Design review of the part built by this model. Coordinates are the model's own, in mm. A direction names the side the tool comes from. Coordinates: 2 decimals unless noted, no trailing zeros. Order: outer loops, then holes, each group sorted by start corner. A loop starts at its lowest first (then second) coordinate and runs counter-clockwise, first axis right, second up. Notation, with made-up numbers: M 63,56.25 L 71,56.25 A20 ccw 71,94.25 Z; hole C 70.25,2 d3. An arc over 180 degrees is marked long. Use CSV: the item, a comma, the result in double quotes.
```python
from build123d import *

# Parameters (mm, degrees)
BOSS_EXTRUDE1_DEPTH = 5.842
SKETCH2_R           = 2.54
BOSS_EXTRUDE2_DEPTH = 2.54
CUT_EXTRUDE1_REACH  = 37.14
SKETCH3_R           = 1.016


with BuildPart() as part:
    # Sketch1 → Boss-Extrude1 (new, symmetric)
    with BuildSketch(Plane.XY):
        Polygon((0, 0), (23.749, 0), (23.749, 16.891), (28.067, 16.891), (28.067, 20.32), (23.749, 20.32), (23.749, 26.162), (0, 26.162), (0, 20.32), (-4.318, 20.32), (-4.318, 16.891), (0, 16.891), align=None)
    extrude(amount=BOSS_EXTRUDE1_DEPTH, both=True)

    # Sketch2 → Boss-Extrude2 (add)
    with BuildSketch(Plane(origin=(0, 26.162, 0), x_dir=(1, 0, 0), z_dir=(0, 1, 0))):
        with Locations((6.0198, 0)):
            Circle(SKETCH2_R)
    extrude(amount=BOSS_EXTRUDE2_DEPTH)

    # Sketch3 → Cut-Extrude1 (cut, up to next)
    with BuildSketch(Plane(origin=(0, 20.32, 0), x_dir=(1, 0, 0), z_dir=(0, 1, 0)), mode=Mode.PRIVATE) as cut_extrude1_sk1:
        with Locations(Location((-2.286, 0, 0), (0, 0, 180))):
            Circle(SKETCH3_R)
    cut_extrude1_tool1 = extrude(cut_extrude1_sk1.sketch, amount=-CUT_EXTRUDE1_REACH, mode=Mode.PRIVATE) & part.part
    # Sketch3 → Cut-Extrude1 (cut, up to next)
    with BuildSketch(Plane(origin=(0, 20.32, 0), x_dir=(1, 0, 0), z_dir=(0, 1, 0)), mode=Mode.PRIVATE) as cut_extrude1_sk2:
        with Locations(Location((-1.778, 3.302, 0), (0, 0, 180))):
            Circle(SKETCH3_R)
    cut_extrude1_tool2 = extrude(cut_extrude1_sk2.sketch, amount=-CUT_EXTRUDE1_REACH, mode=Mode.PRIVATE) & part.part
    # Sketch3 → Cut-Extrude1 (cut, up to next)
    with BuildSketch(Plane(origin=(0, 20.32, 0), x_dir=(1, 0, 0), z_dir=(0, 1, 0)), mode=Mode.PRIVATE) as cut_extrude1_sk3:
        with Locations(Location((-1.778, -3.302, 0), (0, 0, 180))):
            Circle(SKETCH3_R)
    cut_extrude1_tool3 = extrude(cut_extrude1_sk3.sketch, amount=-CUT_EXTRUDE1_REACH, mode=Mode.PRIVATE) & part.part
    # Sketch3 → Cut-Extrude1 (cut, up to next)
    with BuildSketch(Plane(origin=(0, 20.32, 0), x_dir=(1, 0, 0), z_dir=(0, 1, 0)), mode=Mode.PRIVATE) as cut_extrude1_sk4:
        with Locations(Location((25.527, -3.302, 0), (0, 0, 180))):
            Circle(SKETCH3_R)
    cut_extrude1_tool4 = extrude(cut_extrude1_sk4.sketch, amount=-CUT_EXTRUDE1_REACH, mode=Mode.PRIVATE) & part.part
    # Sketch3 → Cut-Extrude1 (cut, up to next)
    with BuildSketch(Plane(origin=(0, 20.32, 0), x_dir=(1, 0, 0), z_dir=(0, 1, 0)), mode=Mode.PRIVATE) as cut_extrude1_sk5:
        with Locations(Location((26.035, 0, 0), (0, 0, 180))):
            Circle(SKETCH3_R)
    cut_extrude1_tool5 = extrude(cut_extrude1_sk5.sketch, amount=-CUT_EXTRUDE1_REACH, mode=Mode.PRIVATE) & part.part
    # Sketch3 → Cut-Extrude1 (cut, up to next)
    with BuildSketch(Plane(origin=(0, 20.32, 0), x_dir=(1, 0, 0), z_dir=(0, 1, 0)), mode=Mode.PRIVATE) as cut_extrude1_sk6:
        with Locations(Location((25.527, 3.302, 0), (0, 0, 180))):
            Circle(SKETCH3_R)
    cut_extrude1_tool6 = extrude(cut_extrude1_sk6.sketch, amount=-CUT_EXTRUDE1_REACH, mode=Mode.PRIVATE) & part.part
    add(cut_extrude1_tool1.solids().sort_by_distance((-2.286, 20.32, 0))[0], mode=Mode.SUBTRACT)
    add(cut_extrude1_tool2.solids().sort_by_distance((-1.778, 20.32, -3.302))[0], mode=Mode.SUBTRACT)
    add(cut_extrude1_tool3.solids().sort_by_distance((-1.778, 20.32, 3.302))[0], mode=Mode.SUBTRACT)
    add(cut_extrude1_tool4.solids().sort_by_distance((25.527, 20.32, 3.302))[0], mode=Mode.SUBTRACT)
    add(cut_extrude1_tool5.solids().sort_by_distance((26.035, 20.32, 0))[0], mode=Mode.SUBTRACT)
    add(cut_extrude1_tool6.solids().sort_by_distance((25.527, 20.32, -3.302))[0], mode=Mode.SUBTRACT)


solid = part.part
```
(1) Add section C-C on x = 23. State the section outline as (y, z) points.
The answers:
outline,"M 0,-5.84 L 26.16,-5.84 L 26.16,5.84 L 0,5.84 Z"
(2) Clearance check with flat-ended pins moving along their axes: P1, Ø1.3, axis at x = -3, z = 0, coming from the +Y side; P2, Ø1.8, axis at y = 24, z = -2.5, coming from the +X side; P3, Ø2.5, axis at x = -1.778, z = 3.302, coming from the -Y side. State where each tip first meets the part, or that it passes through.
The answers:
P1,"stops at y = 20.32"
P2,"stops at x = 23.75"
P3,"stops at y = 16.89"
(3) Wall thickness on probe 1 along X at (y, z) = (20.25, 3); probe 2 along X at (y, z) = (19, -4); probe 3 along Y at (x, z) = (22, 3.5): over which ranges is each line inside the solid? List them lowest first.
The answers:
probe 1,"x = -4.32 to -2.75, -0.81 to 24.56, 26.5 to 28.07"
probe 2,"x = -4.32 to -2.52, -1.04 to 24.79, 26.27 to 28.07"
probe 3,"y = 0 to 26.16"
(4) For faces 4 (the face through (-1, 16.891, 0)), 5 (the face through (0, 23, 0)), 6 (the face through (8.443, 27.414, -0.763)), 7 (the face through (28.067, 19, 0)), 8 (the face through (23.749, 8, 0)), list the 3-axis set-ups (+Z, -Z, +X, -X, +Y, -Y) from which the entire face can be reached by the end or side of a thin tool; tool diameter is ignored.
The answers:
face 4,"+Z, -Z, -X, -Y"
face 5,"+Z, -Z, -X, +Y"
face 6,"+Y"
face 7,"+Z, -Z, +X, +Y, -Y"
face 8,"+Z, -Z, +X, -Y"
(5) Add section A-A on z = 0. State the section outline as (x, y) points.
The answers:
outline,"M -4.32,16.89 L -3.3,16.89 L -3.3,20.32 L -4.32,20.32 Z; M -1.27,16.89 L 0,16.89 L 0,0 L 23.75,0 L 23.75,16.89 L 25.02,16.89 L 25.02,20.32 L 23.75,20.32 L 23.75,26.16 L 8.56,26.16 L 8.56,28.7 L 3.48,28.7 L 3.48,26.16 L 0,26.16 L 0,20.32 L -1.27,20.32 Z; M 27.05,16.89 L 28.07,16.89 L 28.07,20.32 L 27.05,20.32 Z"
(6) The part is to be moulded in two halves that separate along X. For faces 1 (the face through (12, 13, 5.842)), 2 (the face through (23.749, 23, 0)), 3 (the face through (26.54, 18.63, 3.35)), say which applies: pulls with the +X half, pulls with the -X half, needs draft (parallel to the pull), parting line crosses it, or undercut.
The answers:
face 1,"needs draft"
face 2,"pulls with the +X half"
face 3,"undercut"
(7) Add section B-B on y = 14.25. State the section outline as (x, z) points.
The answers:
outline,"M 0,-5.84 L 23.75,-5.84 L 23.75,5.84 L 0,5.84 Z"
